```python
from build123d import *

# Parameters (mm, degrees)
F3_DEPTH = 12
F4_R     = 2.99999
F5_SIZE  = 1.74999


# Not quite as in the source:
# - a fillet or chamfer is up to 0.001 mm smaller than in the source, because OpenCascade refuses the exact size


with BuildPart() as f1:
    # F0 (on Front) → F1 (revolve)
    with BuildSketch(Plane.XZ):
        Polygon((0, 3), (0, 0), (10.75, 0), (10.75, 3), (8.75, 3), (8.75, 7.5), (10.5, 7.5), (8.75, 17), (7.25, 17), (7.25, 3), align=None)
    revolve(axis=Axis((0, 0, 1.5), (0, 0, 1)))

    # F2 (on face) → F3 (cut, through all)
    with BuildSketch(Plane.XY.offset(17)):
        with BuildLine():
            Line((1, -7.1807033082), (1, 7.1807033082))
            ThreePointArc((1, 7.1807033082), (0, 7.25), (-1, 7.1807033082))
            Line((-1, 7.1807033082), (-1, -7.1807033082))
            ThreePointArc((-1, -7.1807033082), (0, -7.25), (1, -7.1807033082))
        make_face()
        with BuildLine():
            Line((1, 7.1807033082), (1, 8.6926693254))
            ThreePointArc((1, 8.6926693254), (0, 8.75), (-1, 8.6926693254))
            Line((-1, 8.6926693254), (-1, 7.1807033082))
            ThreePointArc((-1, 7.1807033082), (0, 7.25), (1, 7.1807033082))
        make_face()
        with BuildLine():
            Line((-1, -7.1807033082), (-1, -8.6926693254))
            ThreePointArc((-1, -8.6926693254), (0, -8.75), (1, -8.6926693254))
            Line((1, -8.6926693254), (1, -7.1807033082))
            ThreePointArc((1, -7.1807033082), (0, -7.25), (-1, -7.1807033082))
        make_face()
        with BuildLine():
            ThreePointArc((1, -8.6926693254), (0, -8.75), (-1, -8.6926693254))
            Line((-1, -8.6926693254), (-1, -25))
            Line((-1, -25), (1, -25))
            Line((1, -25), (1, -8.6926693254))
        make_face()
        with BuildLine():
            Line((1, 8.6926693254), (1, 25))
            Line((1, 25), (-1, 25))
            Line((-1, 25), (-1, 8.6926693254))
            ThreePointArc((-1, 8.6926693254), (0, 8.75), (1, 8.6926693254))
        make_face()
    extrude(amount=-F3_DEPTH, mode=Mode.SUBTRACT)

    # F4 (radius 3 in the source; OpenCascade refuses exactly that, so slightly less here)
    f4_edges = [f1.edges().sort_by_distance(p)[0] for p in [
        (-10.75, 0, 0),
    ]]
    fillet(f4_edges, radius=F4_R)

    # F5 (size 1.75 in the source; OpenCascade refuses exactly that, so slightly less here)
    f5_edges = [f1.edges().sort_by_distance(p)[0] for p in [
        (-8.75, 0, 7.5),
        (6.531175, 5.822907, 7.5),
        (6.531175, -5.822907, 7.5),
    ]]
    chamfer(f5_edges, length=F5_SIZE)


solid = f1.part
```
Could you check a few things on this model? Use its own coordinates, in mm. A direction names the side the tool comes from. Coordinates: 2 decimals unless noted, no trailing zeros. Order: outer loops, then holes, each group sorted by start corner. A loop starts at its lowest first (then second) coordinate and runs counter-clockwise, first axis right, second up. Notation, with made-up numbers: M -14,76.5 L 13,76.5 A21 cw 13,114.5 Z; hole C -9,82 d10. An arc over 180 degrees is marked long. Use a Markdown table: item, result. Add a question column.
Q1. If I drill on L1, parallel to Z at x = -0.75, y = -1.25; L2, parallel to Y at x = -6.25, z = 8.5; L3, parallel to X at y = -7.25, z = 10, over which ranges is the centre line in solid material (lowest first)?
Q2. I want a section at C-C on z = 11.25. List the corners of the cut face in (x, y) for me, then the cut area to 3 significant figures.
Q3. I'm going to push flat-ended pins straight in: pin 1 (1 mm diameter, centred on x = -1, y = -0.5, fed in from -Z); pin 2 (1 mm diameter, centred on y = -9, z = 12, fed in from -X); pin 3 (3 mm diameter, centred on x = -3.5, z = 11, fed in from -Y); pin 4 (6 mm diameter, centred on x = -2, y = 0, fed in from +Z). Where does each tip first touch, or does it pass through?
Q4. We'd pull the mould along Z, two halves only. Please class faces 5 (the flat face through (2, -9, 3)), 6 (the flat face through (0, 0, 0)), 7 (the flat face through (0, 0, 3)), 8 (the conical face through (-9, 0, 6)): pulls with the +Z half, pulls with the -Z half, needs draft (parallel to the pull), parting line crosses it, or undercut.
Q5. Which directions (+Z, -Z, +X, -X, +Y, -Y) give clear straight access to the entire face, cutting with the end or side of a thin tool? Please do faces 1 (the conical face through (9, 0, 6)), 2 (the flat face through (-1, 8, 11)), 3 (the cylindrical face through (3.35, -6.43, 9.9)), 4 (the flat face through (-7.5, -0.6, 17)).
Checked values:
| question | item | result |
|---|---|---|
| 1 | L1 | 0 to 3 |
| 1 | L2 | -8.21 to -3.67, 3.67 to 8.21 |
| 1 | L3 | -6.94 to -1, 1 to 6.94 |
| 2 | outline | M -1,-9.76 L -1,-7.18 A7.25 cw -1,7.18 L -1,9.76 A9.81 ccw Z; M 1,-9.76 A9.81 ccw 1,9.76 L 1,7.18 A7.25 cw 1,-7.18 Z |
| 2 | area | 127 mm² |
| 3 | pin 1 | z = 0 |
| 3 | pin 2 | x = -4.63 |
| 3 | pin 3 | y = -9.75 |
| 3 | pin 4 | z = 3 |
| 4 | face 5 | undercut |
| 4 | face 6 | pulls with the -Z half |
| 4 | face 7 | pulls with the +Z half |
| 4 | face 8 | undercut |
| 5 | face 1 | +X |
| 5 | face 2 | +Z, +Y, -Y |
| 5 | face 3 | +Z |
| 5 | face 4 | +Z, +X, -X, +Y, -Y |
